```python
from build123d import *

# Parameters (mm, degrees)
SKETCH1_W           = 80
SKETCH1_H           = 80
BOSS_EXTRUDE1_DEPTH = 16
SKETCH2_R           = 35
CUT_EXTRUDE1_DEPTH  = 17


with BuildPart() as part:
    # Sketch1 → Boss-Extrude1 (new body)
    with BuildSketch(Plane(origin=(0, 0, 0), x_dir=(1, 0, 0), z_dir=(0, 1, 0))):
        Rectangle(SKETCH1_W, SKETCH1_H)
    extrude(amount=BOSS_EXTRUDE1_DEPTH)

    # Sketch2 → Cut-Extrude1 (cut, through all)
    with BuildSketch(Plane.XZ):
        Circle(SKETCH2_R)
    extrude(amount=-CUT_EXTRUDE1_DEPTH, mode=Mode.SUBTRACT)


solid = part.part
```
Source: CAD feature listing. Evaluate the final solid. Frame: model axes, mm. Coordinates: 2 decimals unless noted, no trailing zeros. Write each loop counter-clockwise with the first axis right and the second up, starting at its lowest first coordinate (ties: lowest second). Pieces come first, ordered by that corner, then holes. Notation, with made-up numbers: (31.25, -9.5) - (75.25, -9.5) arc R21 cw to (75.25, 21.5) - close; hole circle Ø6 at (23.5, 45). An arc over 180 degrees is marked (long way). Answer as a JSON object with one key per item and string values.
Q1. Section query A-A, the plane x = 0. Output: boundary loops of the cut face in (y, z), plus the area to 3 significant figures.
Ans:
{"outline": "(0, -40) - (16, -40) - (16, -35) - (0, -35) - close; (0, 35) - (16, 35) - (16, 40) - (0, 40) - close", "area": "160 mm2"}
Q2. Section query C-C, the plane y = 10.25. Output: boundary loops of the cut face in (x, z).
Ans:
{"outline": "(-40, -40) - (40, -40) - (40, 40) - (-40, 40) - close; hole circle Ø70 at (0, 0)"}
Q3. Draft query along X for faces 1 (the flat face through (-1, 8, -40)), 2 (the flat face through (-40, 8, 1)), 3 (the cylindrical face through (-28, 8, -21)). Return one class per face: released by +X, released by -X, zero draft, split by the parting line, or undercut.
Ans:
{"face 1": "zero draft", "face 2": "released by -X", "face 3": "undercut"}
Q4. Material intervals for line 1 (Z direction, x = 0, y = 7.75); line 2 (X direction, y = 13.25, z = -10.5); line 3 (X direction, y = 8.25, z = -12), sorted ascending. Write a range as [from, to].
Ans:
{"line 1": "z = [-40, -35], [35, 40]", "line 2": "x = [-40, -33.39], [33.39, 40]", "line 3": "x = [-40, -32.88], [32.88, 40]"}
Q5. Section query B-B, the plane z = 0. Output: boundary loops of the cut face in (x, y).
Ans:
{"outline": "(-40, 0) - (-35, 0) - (-35, 16) - (-40, 16) - close; (35, 0) - (40, 0) - (40, 16) - (35, 16) - close"}
